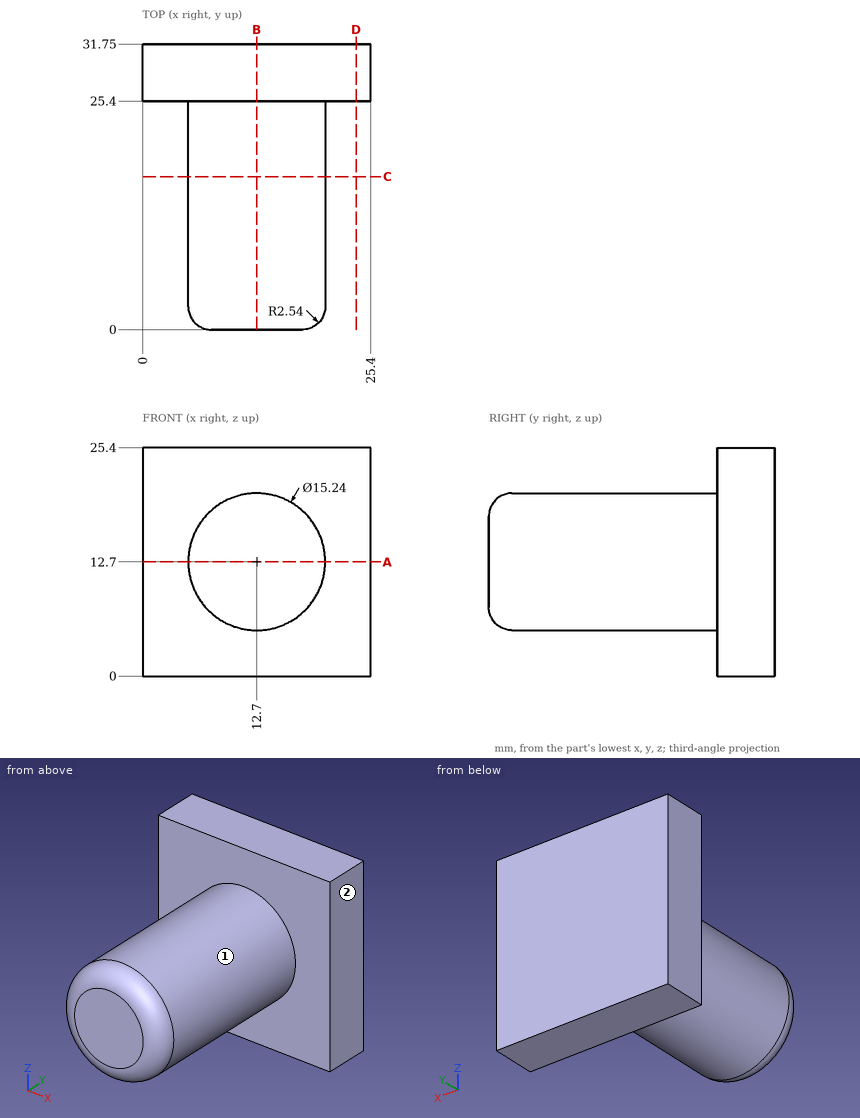
Can you work these out from the drawing? Everything is in mm from the part's minimum corner. A direction names the side the tool comes from. Give positions to 0.01 mm unless a question says otherwise; leave off trailing zeros. Order: outer loops, then holes, each group sorted by start corner. A loop starts at its lowest first (then second) coordinate and runs counter-clockwise, first axis right, second up.
Item 1: I'm going to push flat-ended pins straight in: pin 1 (3 mm diameter, centred on x = 18, z = 22, fed in from -Y); pin 2 (8 mm diameter, centred on x = 22.5, y = 8.5, fed in from +Z); pin 3 (3 mm diameter, centred on x = 5.5, y = 20, fed in from -Z). Where does each tip first touch, or does it pass through?
Item 2: For the marked faces 1 and 2, which set-ups out of +Z, -Z, +X, -X, +Y, -Y let a thin tool reach every point of the face, with its end or its side?
Item 3: If we section it at C-C, the plane y = 17: Write out the boundary of the cut face in (x, z).
Item 4: If we section it at A-A, the plane z = 12.7: Write out the boundary of the cut face in (x, y).
Item 5: If we section it at D-D, the plane x = 23.75: Write out the boundary of the cut face in (y, z), plus the area to 3 significant figures.
Item 6: If we section it at B-B, the plane x = 12.7: Write out the boundary of the cut face in (y, z).
Item 7: I need wall thicknesses on line 1 (Y direction, x = 5.75, z = 9); line 2 (Z direction, x = 12.5, y = 22.5); line 3 (X direction, y = 7, z = 10). Which ranges of each line are inside material? Lowest first, please.
Values:
1. pin 1: stops at y = 25.4
1. pin 2: stops at z = 17.64
1. pin 3: stops at z = 7.64
2. face 1: -Y
2. face 2: +Z, -Z, +X, +Y, -Y
3. outline: circle Ø15.24 at (12.7, 12.7)
4. outline: (0, 25.4) - (5.08, 25.4) - (5.08, 2.54) arc R2.54 ccw to (7.62, 0) - (17.78, 0) arc R2.54 ccw to (20.32, 2.54) - (20.32, 25.4) - (25.4, 25.4) - (25.4, 31.75) - (0, 31.75) - close
5. outline: (25.4, 0) - (31.75, 0) - (31.75, 25.4) - (25.4, 25.4) - close
5. area: 161 mm2
6. outline: (0, 7.62) arc R2.54 ccw to (2.54, 5.08) - (25.4, 5.08) - (25.4, 0) - (31.75, 0) - (31.75, 25.4) - (25.4, 25.4) - (25.4, 20.32) - (2.54, 20.32) arc R2.54 ccw to (0, 17.78) - close
7. line 1: y = 25.4 to 31.75
7. line 2: z = 5.08 to 20.32
7. line 3: x = 5.57 to 19.83
